Geometry check sheet. Reference: the model listing, model coordinates, mm. Face numbers are marked on the shaded views. A direction names the side the tool comes from. Coordinates: 2 decimals unless noted, no trailing zeros. Order: outer loops, then holes, each group sorted by start corner. A loop starts at its lowest first (then second) coordinate and runs counter-clockwise, first axis right, second up. Notation, with made-up numbers: (-30, -29) - (22, -29) arc R21 ccw to (22, 8) - close; hole circle Ø2 at (63.5, 36). An arc over 180 degrees is marked (long way). Return JSON: item names as keys, results as strings. Group by question number.
Item 1: Section check B-B on x = 0. Enter the section's corners in (y, z), then the cut area to 3 significant figures.
Item 2: Section check C-C on y = 2.25. Enter the section's corners in (x, z), then the cut area to 3 significant figures.
Item 3: Tool access check on the marked faces 1 and 2. Record the directions out of +Z, -Z, +X, -X, +Y, -Y that give a thin tool (end or side, any length) a straight path to the whole face; none if there is none.
Item 4: Draft check along Z on the marked faces 3, 4 and 5. Enter one of: pulls with the +Z half, pulls with the -Z half, needs draft (parallel to the pull), parting line crosses it, or undercut.
Item 5: Gauge pin test, flat end, axial feed: pin 1 (3 mm diameter, centred on y = 3, z = 2.5, fed in from +X). Record the tip position at first contact, or that the pin passes through.
Item 6: Section check D-D on z = -2.25. Enter the section's corners in (x, y).
Item 7: Section check A-A on z = 0. Enter the section's corners in (x, y).
Item 8: Scan lines: probe 1 along X at (y, z) = (1.6, 0); probe 2 along Z at (x, y) = (0.75, 4.3); probe 3 along X at (y, z) = (4.8, -0.75). Record each from-to range of solid material in increasing order.
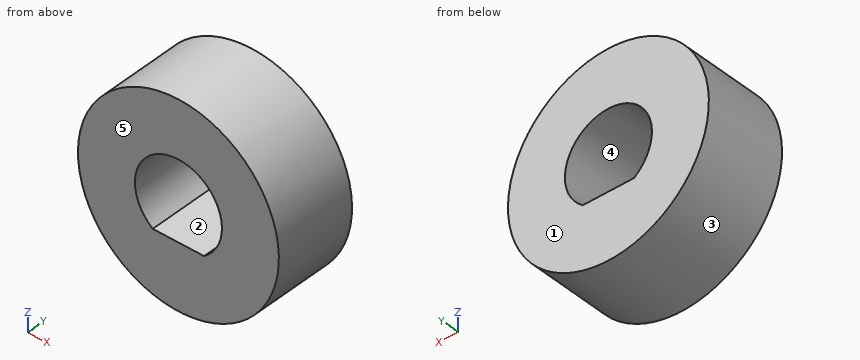
from build123d import *

# Parameters (mm, degrees)
SKETCH1_R           = 6
BOSS_EXTRUDE1_DEPTH = 5
BOSS_EXTRUDE2_START = -5
BOSS_EXTRUDE2_DEPTH = 5
CUT_EXTRUDE1_DEPTH  = 5


with BuildPart() as part:
    # Sketch1 → Boss-Extrude1 (new body)
    with BuildSketch(Plane(origin=(0, 0, 0), x_dir=(1, 0, 0), z_dir=(0, 1, 0))):
        with Locations(Location((0, 0, 0), (0, 0, 270))):
            Circle(SKETCH1_R)
        with BuildLine():
            ThreePointArc((-1.549193338, 2.15), (0, -2.65), (1.549193338, 2.15))
            Line((1.549193338, 2.15), (-1.549193338, 2.15))
        make_face(mode=Mode.SUBTRACT)
    extrude(amount=BOSS_EXTRUDE1_DEPTH)

    # Sketch2 → Boss-Extrude2 (add)
    with BuildSketch(Plane(origin=(0, 5, 0), x_dir=(1, 0, 0), z_dir=(0, 1, 0)).offset(BOSS_EXTRUDE2_START)):
        with BuildLine():
            Line((1.549193338, 2.15), (-1.549193338, 2.15))
            ThreePointArc((-1.549193338, 2.15), (0, -2.65), (1.549193338, 2.15))
        make_face()
        with BuildLine():
            Line((1.526433752, 2.08), (-1.526433752, 2.08))
            ThreePointArc((-1.526433752, 2.08), (0, -2.58), (1.526433752, 2.08))
        make_face(mode=Mode.SUBTRACT)
    extrude(amount=BOSS_EXTRUDE2_DEPTH)

    # Sketch3 → Cut-Extrude1 (cut)
    with BuildSketch(Plane(origin=(0, 5, 0), x_dir=(1, 0, 0), z_dir=(0, 1, 0))):
        with BuildLine():
            Line((1.532970972, 2.1), (-1.532970972, 2.1))
            ThreePointArc((-1.532970972, 2.1), (0, -2.6), (1.532970972, 2.1))
        make_face()
    extrude(amount=-CUT_EXTRUDE1_DEPTH, mode=Mode.SUBTRACT)


solid = part.part
Computed:
{
 "1": {"outline": "(0, -6) - (5, -6) - (5, -2.1) - (0, -2.1) - close; (0, 2.6) - (5, 2.6) - (5, 6) - (0, 6) - close", "area": "36.5 mm²"},
 "2": {"outline": "circle Ø12 at (0, 0); hole (-1.53, -2.1) - (1.53, -2.1) arc R2.6 ccw (long way) to start", "area": "92.9 mm²"},
 "3": {"face 1": "+Z, -Z, +X, -X, +Y", "face 2": "+Y, -Y"},
 "4": {"face 3": "parting line crosses it", "face 4": "undercut", "face 5": "needs draft"},
 "5": {"pin 1": "stops at x = 5.92"},
 "6": {"outline": "(-5.56, 0) - (5.56, 0) - (5.56, 5) - (-5.56, 5) - close"},
 "7": {"outline": "(-6, 0) - (-2.6, 0) - (-2.6, 5) - (-6, 5) - close; (2.6, 0) - (6, 0) - (6, 5) - (2.6, 5) - close"},
 "8": {"probe 1": "x = -6 to -2.6, 2.6 to 6", "probe 2": "z = -5.95 to -2.1, 2.49 to 5.95", "probe 3": "x = -5.95 to -2.49, 2.49 to 5.95"}
}
